from build123d import *

# Parameters (mm, degrees)
PAD_DEPTH          = 3
POLARPATTERN_COUNT = 3
CHAMFER_SIZE       = 1.5


with BuildPart() as part:
    # Sketch → Revolution (revolve)
    with BuildSketch(Plane.XZ):
        Polygon((5, 0), (8.5, 0), (8.5, 9), (7.5, 9), (7.5, 2), (5, 2), align=None)
    revolve(axis=Axis((0, 0, 0), (0, 0, 1)))

    # Sketch001 → Pad (new body)
    with BuildSketch(Plane.XY):
        with BuildLine():
            ThreePointArc((-4.7140452079, 5.8333333333), (0, 2.5), (4.7140452079, 5.8333333333))
            ThreePointArc((4.7140452079, 5.8333333333), (0, 7.5), (-4.7140452079, 5.8333333333))
        make_face()
    pad = extrude(amount=PAD_DEPTH)

    # PolarPattern: Pad ×3 about axis
    polarpattern_axis = Axis((0, 0, 0), (0, 0, 1))
    for i in range(1, POLARPATTERN_COUNT):
        add(pad.rotate(polarpattern_axis, i * 360 / POLARPATTERN_COUNT))

    # Chamfer
    chamfer_edges = [part.edges().sort_by_distance(p)[0] for p in [
        (-8.5, 0, 0),
    ]]
    chamfer(chamfer_edges, length=CHAMFER_SIZE)


solid = part.part
Check sheet for the modelled part. Datum: model origin and axes. Units: mm. A direction names the side the tool comes from. Give positions to 0.01 mm unless a question says otherwise; leave off trailing zeros. Write each loop counter-clockwise with the first axis right and the second up, starting at its lowest first coordinate (ties: lowest second). Pieces come first, ordered by that corner, then holes. Notation, with made-up numbers: (-14.75, 82.5) -> (27.25, 82.5) arc R32 ccw to (27.25, 117.5) -> close; hole circle Ø10 at (78, -23.5). An arc over 180 degrees is marked (long way). One line per item, written item: value. Start each with the question number.
Item 1: Gauge pin test, flat ends, axial feed: pin 1 (2.5 mm diameter, centred on x = 0.5, y = 4, fed in from +Z); pin 2 (1 mm diameter, centred on x = 6, z = 1.5, fed in from -Y); pin 3 (1.4 mm diameter, centred on x = -0.5, y = -5.5, fed in from +Z). Record the tip position at first contact, or that the pin passes through.
Item 2: Section check B-B on y = 0. Record the cut outline in (x, z), then the cut area to 3 significant figures.
Item 3: Material ranges on probe 1 along Y at (x, z) = (0, 4.25); probe 2 along Z at (x, y) = (0.25, 4.25); probe 3 along X at (y, z) = (-0.75, 2.25), recorded low to high. Write a range as from..to.
Item 4: Section check C-C on z = 5.25. Record the cut outline in (x, y), then the cut area to 3 significant figures.
Item 5: Tool access check on faces 1 (the cylindrical face through (4.34, 2.48, 0.99)), 2 (the flat face through (0, 3, 0)), 3 (the flat face through (4, -2, 3)). Record the directions out of +Z, -Z, +X, -X, +Y, -Y that give a thin tool (end or side, any length) a straight path to the whole face; none if there is none.
Item 6: Section check A-A on x = 0. Record the cut outline in (y, z), then the cut area to 4 significant figures.
Results list:
1. pin 1: z = 3
1. pin 2: y = -6.48
1. pin 3: z = 2
2. outline: (-8.5, 1.5) -> (-7, 0) -> (-3.19, 0) -> (-3.19, 3) -> (-7.5, 3) -> (-7.5, 9) -> (-8.5, 9) -> close; (3.19, 0) -> (7, 0) -> (8.5, 1.5) -> (8.5, 9) -> (7.5, 9) -> (7.5, 3) -> (3.19, 3) -> close
2. area: 41.6 mm²
3. probe 1: -8.5..-7.5, 7.5..8.5
3. probe 2: 0..3
3. probe 3: -8.47..-2.5, 2.5..8.47
4. outline: circle Ø17 at (0, 0); hole circle Ø15 at (0, 0)
4. area: 50.3 mm²
5. face 1: +Z, -Z
5. face 2: -Z, +X, -X, +Y, -Y
5. face 3: +Z
6. outline: (-8.5, 1.5) -> (-7, 0) -> (-5, 0) -> (-5, 2) -> (-7.5, 2) -> (-7.5, 9) -> (-8.5, 9) -> close; (2.5, 0) -> (7, 0) -> (8.5, 1.5) -> (8.5, 9) -> (7.5, 9) -> (7.5, 3) -> (2.5, 3) -> close
6. area: 35.75 mm²
